Input: part model. Units: mm. Frame: model coordinates. A direction names the side the tool comes from. Give positions to 0.01 mm unless a question says otherwise; leave off trailing zeros. Loops run counter-clockwise (first coordinate to the right, second up) from the corner with the lowest first, then second, coordinate; pieces in that order, holes last. Notation, with made-up numbers: M -36,77.25 L 12,77.25 A12 ccw 12,92.25 Z; hole C 49,9.5 d1. An arc over 180 degrees is marked long. One line per item, written item: value. Start each with the question number.
(1) Access query for faces 1 (the cylindrical face through (3.905, 175.371, 0.867)), 2 (the flat face through (1, 193.5, 1)). Directions: +Z, -Z, +X, -X, +Y, -Y. A direction counts if a zero-diameter tool reaches every point of the face in a straight line with its end or side. Return the directions, or none.
(2) Pin query (flat end, axial travel): P1, Ø5, axis at x = 4, y = 75, coming from the -Z side; P2, Ø4, axis at x = 2.5, y = 22, coming from the -Z side. Return the tip coordinate at first contact, or that it passes through.
(3) Section A-A on y = 134. Output: boundary loops of the cut face in (x, z), plus the area to 3 significant figures.
(4) Ray query, line 1 along X through (y, z) = (158.5, 0); line 2 along Y through (x, z) = (-3.75, 1.5); line 3 along Z through (x, y) = (0.75, 20.5). Return the intervals inside material, ascending. Write a range as from..to.
```python
from build123d import *

# Parameters (mm, degrees)
DIAM_TRE_DU_PER_AGE_3_0_3_1_D     = 3
DIAM_TRE_DU_PER_AGE_3_0_3_1_DEPTH = 40
DIAM_TRE_DU_PER_AGE_3_0_3_1_TIP   = 0.901290929
CHANFREIN1_SIZE                   = 2
CHANFREIN1_SIZE2                  = 7.464101615


with BuildPart() as part:
    # Esquisse1 → Révolution1 (revolve)
    with BuildSketch(Plane.XY, mode=Mode.PRIVATE) as r_volution1_sk:
        Polygon((1, -35), (1, 193.5), (4, 193.5), (4, 165), (5, 165), (5, 20), (5, -35), align=None)
    revolve(r_volution1_sk.sketch.rotate(Axis((0, 0, 0), (0, 1, 0)), 90), axis=Axis((0, 0, 0), (0, 1, 0)))

    # Diamètre du perçage Ø3.0 (3)1
    with Locations(Plane(origin=(0, -35, 0), x_dir=(-1, 0, 0), z_dir=(0, -1, 0))):
        with Locations((0, 0)):
            Hole(DIAM_TRE_DU_PER_AGE_3_0_3_1_D / 2, depth=DIAM_TRE_DU_PER_AGE_3_0_3_1_DEPTH)
            with Locations((0, 0, -(DIAM_TRE_DU_PER_AGE_3_0_3_1_DEPTH + DIAM_TRE_DU_PER_AGE_3_0_3_1_TIP / 2))):  # 118° drill point
                Cone(0, DIAM_TRE_DU_PER_AGE_3_0_3_1_D / 2, DIAM_TRE_DU_PER_AGE_3_0_3_1_TIP, mode=Mode.SUBTRACT)

    # Chanfrein1
    chanfrein1_edges = [part.edges().sort_by_distance(p)[0] for p in [
        (0, 193.5, 4),
    ]]
    chanfrein1_side = [part.faces().sort_by_distance(p)[0] for p in [
        (0, 193.5, 1.113137085),
    ]]
    chamfer(chanfrein1_edges, length=CHANFREIN1_SIZE, length2=CHANFREIN1_SIZE2, reference=chanfrein1_side[0])


solid = part.part
```
Output values:
1. face 1: +Y
1. face 2: +Z, -Z, +X, -X, +Y
2. P1: stops at z = -4.77
2. P2: stops at z = -4.97
3. outline: C 0,0 d10; hole C 0,0 d2
3. area: 75.4 mm²
4. line 1: x = -5..-1, 1..5
4. line 2: y = -35..165
4. line 3: z = -4.94..-0.66, 0.66..4.94
